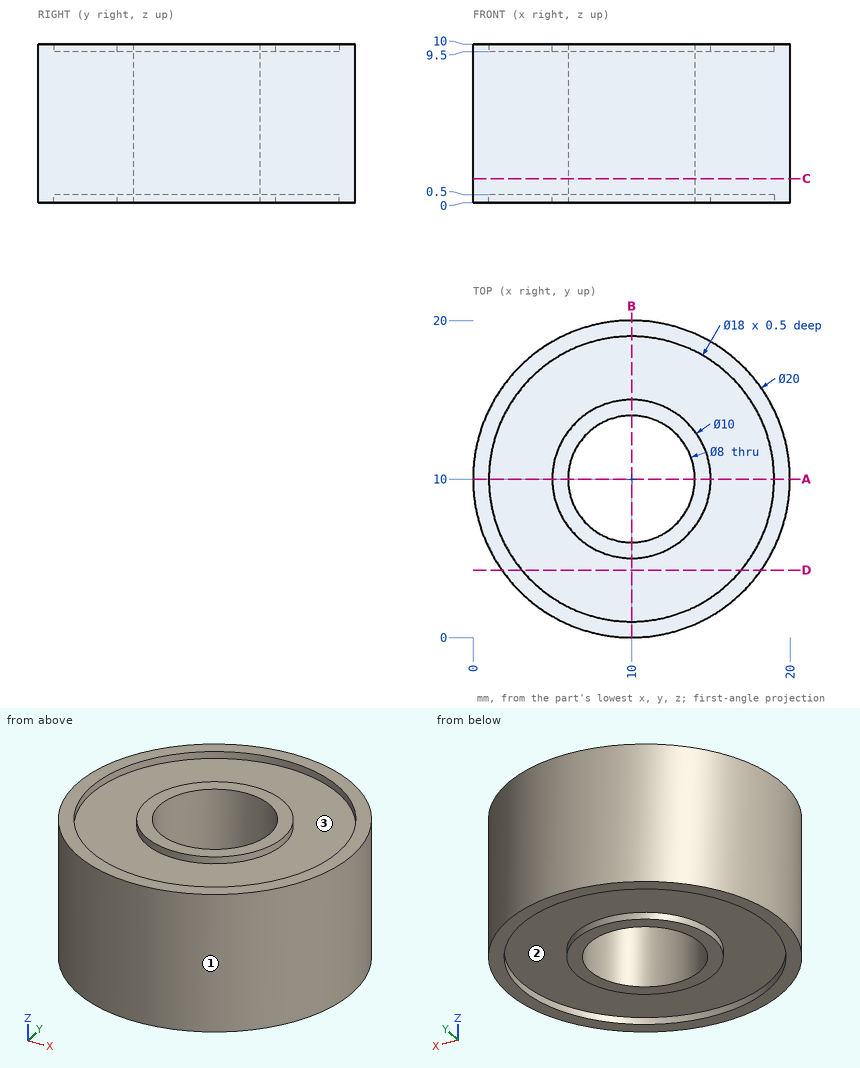
Can you work these out from the drawing? Everything is in mm from the part's minimum corner. Give positions to 0.01 mm unless a question says otherwise; leave off trailing zeros. Loops run counter-clockwise (first coordinate to the right, second up) from the corner with the lowest first, then second, coordinate; pieces in that order, holes last. Notation, with made-up numbers: (50.25, -9) -> (59.25, -9) arc R18 ccw to (59.25, 1) -> close; hole circle Ø3 at (38.5, 75.5). An arc over 180 degrees is marked (long way). Return JSON: item names as keys, results as strings.
Q1. For pin 1 Ø5 at (x, y) = (10, 10) entering from -Z; pin 2 Ø2 at (x, y) = (4.5, 12.5) entering from -Z; pin 3 Ø1 at (x, z) = (17, 8) entering from -Y, each with a flat end and sliding along its axis, tell me the tip position at first contact or that it passes through.
Checks:
{"pin 1": "passes through", "pin 2": "stops at z = 0.5", "pin 3": "stops at y = 2.4"}
Q2. I want a section at C-C, the plane z = 1.5. List the corners of the cut face in (x, y) for me.
Checks:
{"outline": "circle Ø20 at (10, 10); hole circle Ø8 at (10, 10)"}
Q3. I want a section at A-A, the plane y = 10. List the corners of the cut face in (x, z) for me.
Checks:
{"outline": "(0, 0) -> (1, 0) -> (1, 0.5) -> (5, 0.5) -> (5, 0) -> (6, 0) -> (6, 10) -> (5, 10) -> (5, 9.5) -> (1, 9.5) -> (1, 10) -> (0, 10) -> close; (14, 0) -> (15, 0) -> (15, 0.5) -> (19, 0.5) -> (19, 0) -> (20, 0) -> (20, 10) -> (19, 10) -> (19, 9.5) -> (15, 9.5) -> (15, 10) -> (14, 10) -> close"}
Q4. I want a section at D-D, the plane y = 4.25. List the corners of the cut face in (x, z) for me.
Checks:
{"outline": "(1.82, 0) -> (3.08, 0) -> (3.08, 0.5) -> (16.92, 0.5) -> (16.92, 0) -> (18.18, 0) -> (18.18, 10) -> (16.92, 10) -> (16.92, 9.5) -> (3.08, 9.5) -> (3.08, 10) -> (1.82, 10) -> close"}
Q5. We'd pull the mould along X, two halves only. Please class the marked faces 1, 2 and 3: released by +X, released by -X, zero draft, split by the parting line, or undercut.
Checks:
{"face 1": "split by the parting line", "face 2": "undercut", "face 3": "undercut"}
Q6. I need wall thicknesses on probe 1 along Y at (x, z) = (10, 9.7); probe 2 along Y at (x, z) = (10, 2); probe 3 along Y at (x, z) = (6.5, 9.75). Which ranges of each line are inside material? Lowest first, please.
Checks:
{"probe 1": "y = 0 to 1, 5 to 6, 14 to 15, 19 to 20", "probe 2": "y = 0 to 6, 14 to 20", "probe 3": "y = 0.63 to 1.71, 6.43 to 8.06, 11.94 to 13.57, 18.29 to 19.37"}
